Autodesk Inventor part; units mm, degrees
ref_plane "YZ Plane" through (0, 0, 0) normal (1, 0, 0) x (0, 1, 0)
ref_plane "XZ Plane" through (0, 0, 0) normal (0, 1, 0) x (-1, 0, 0)
ref_plane "XY Plane" through (0, 0, 0) normal (0, 0, 1) x (1, 0, 0)
sketch "Sketch1" plane through (0, 0, 0) normal (0, 0, 1) x (1, 0, 0)
  circle A0 centre (0, 0) radius 11.5
  circle A1 centre (0, 0) radius 1.65
  line L0 (-11.5, 0) -> (-11.5, -5)
  line L1 (-11.5, 0) -> (-11.5, 5)
  line L2 (-11.5, 5) -> (-10.3562, 5)
  line L3 (-11.5, -5) -> (-10.3562, -5)
  line L4 (11.5, 0) -> (11.5, 5)
  line L5 (11.5, 5) -> (10.3562, 5)
  line L6 (11.5, 0) -> (11.5, -5)
  line L7 (11.5, -5) -> (10.3562, -5)
  line L8 (-67.75, 0) -> (-67.75, 5)
  line L9 (-67.75, 5) -> (-11.5, 5)
  line L10 (-67.75, 0) -> (-67.75, -5)
  line L11 (-67.75, -5) -> (-11.5, -5)
  line L12 (67.75, -5) -> (67.75, 5)
  line L13 (67.75, 5) -> (11.5, 5)
  line L14 (11.5, -5) -> (67.75, -5)
  line L15 (67.75, -5) -> (71.75, -5)
  line L16 (71.75, -5) -> (71.75, 5)
  line L17 (71.75, 5) -> (67.75, 5)
  line L18 (-67.75, -5) -> (-71.75, -5)
  line L19 (-71.75, -5) -> (-71.75, 5)
  line L20 (-71.75, 5) -> (-67.75, 5)
  line L21 (0, 11.5) -> (-71.75, 11.5)
  line L22 (-71.75, 11.5) -> (-71.75, 5)
  line L23 (-71.75, -5) -> (-71.75, -11.5)
  line L24 (-71.75, -11.5) -> (0, -11.5)
  line L25 (0, -11.5) -> (71.75, -11.5)
  line L26 (71.75, -11.5) -> (71.75, -5)
  line L27 (71.75, 5) -> (71.75, 11.5)
  line L28 (0, 11.5) -> (71.75, 11.5)
  line L29 (67.75, 5) -> (67.75, 11.5)
  line L30 (67.75, 11.5) -> (63.75, 11.5)
  line L31 (63.75, 11.5) -> (63.75, -11.5)
  line L32 (-71.75, -11.5) -> (-63.75, -11.5)
  line L33 (-63.75, -11.5) -> (-63.75, 11.5)
  line L34 (-67.75, -11.5) -> (-75.75, -11.5)
  line L35 (-75.75, -11.5) -> (-75.75, 11.5)
  line L36 (-75.75, 11.5) -> (-67.75, 11.5)
  line L37 (-67.75, 11.5) -> (-67.75, -11.5)
  line L38 (67.75, 11.5) -> (75.75, 11.5)
  line L39 (75.75, 11.5) -> (75.75, -11.5)
  line L40 (75.75, -11.5) -> (67.75, -11.5)
  line L41 (67.75, -11.5) -> (67.75, 11.5)
  dimension "d0" = 23
  dimension "d1" = 3.3
  dimension "d4" = 5
  dimension "d5" = 5
  dimension "d6" = 5
  dimension "d7" = 5
  dimension "d12" = 4
  dimension "d13" = 4
  dimension "d20" = 4
  dimension "d21" = 8
  dimension "d24" = 8
  dimension "d25" = 8
extrude "Extrusion1" add sketch "Sketch1" along normal blind 8
extrude "Extrusion2" add sketch "Sketch1" against normal blind 80 contours L17 L16 L15 L12 | L29 L28 L27 L17 | L15 L26 L25 L41 | L37 L20 L22 L21 | L24 L23 L18 L37 | L27 L38 L39 L40 L26 L16 | L22 L19 L23 L34 L35 L36 | L8 L10 L18 L19 L20
sketch "Sketch4" plane through (75.75, -11.5, 8) normal (1, 0, 0) x (0, 0, -1)
  circle A0 centre (79.1099, 11.5) radius 1.75
  point P0 (8, 11.5)
  dimension "d26" = 3.5
extrude "Extrusion5" cut sketch "Sketch4" against normal blind 800
properties part number "Sensor houder" material "ABS Plastic"
Geometry check sheet. Reference: the model listing, model coordinates, mm. A direction names the side the tool comes from. Give positions to 0.01 mm unless a question says otherwise; leave off trailing zeros. Write each loop counter-clockwise with the first axis right and the second up, starting at its lowest first coordinate (ties: lowest second). Pieces come first, ordered by that corner, then holes. Notation, with made-up numbers: M -1.75,83 L 3.25,83 A25 ccw 3.25,119 Z; hole C 8,52.25 d1. An arc over 180 degrees is marked long. Answer as CSV lines item,"result". Start each with the question number.
Q1. Section check B-B, the plane x = 0. Record the cut outline in (y, z).
Q2. Section check A-A, the plane z = -63. Record the cut outline in (x, y).
Q3. Release check for a two-part mould opening along Y. For faces 3 (the face through (67.75, 0, -39)), 4 (the face through (0, -11.5, 3)), 5 (the face through (-71.69, 0.08, -69.36)) record: pulls with the +Y half, pulls with the -Y half, needs draft (parallel to the pull), parting line crosses it, or undercut.
Q4. Section check D-D, the plane y = -9.75. Record the cut outline in (x, z).
Q5. Go/stop test with flat-tipped pins: pin 1 (2 mm diameter, centred on y = 0, z = -71.11, fed in from +X); pin 2 (5 mm diameter, centred on x = -29.5, y = 2.5, fed in from -Z). Record where each tip stops, or that it passes through.
Q6. Material ranges on L1, parallel to X at y = 6.25, z = -37.5; L2, parallel to Y at x = 0, z = 6; L3, parallel to Z at x = -15, y = -2, recorded low to high.
Q7. Section check C-C, the plane y = 0. Record the cut outline in (x, z).
Q8. Tool access check on faces 1 (the face through (-72, 0, -80)), 2 (the face through (-1, 3, 0)). Record the directions out of +Z, -Z, +X, -X, +Y, -Y that give a thin tool (end or side, any length) a straight path to the whole face; none if there is none.
Geometry says:
1,outline,"M -11.5,0 L -1.65,0 L -1.65,8 L -11.5,8 Z; M 1.65,0 L 11.5,0 L 11.5,8 L 1.65,8 Z"
2,outline,"M -75.75,-11.5 L -67.75,-11.5 L -67.75,11.5 L -75.75,11.5 Z; M 67.75,-11.5 L 75.75,-11.5 L 75.75,11.5 L 67.75,11.5 Z"
3,face 3,"needs draft"
3,face 4,"pulls with the -Y half"
3,face 5,"undercut"
4,outline,"M -75.75,-80 L -67.75,-80 L -67.75,0 L 67.75,0 L 67.75,-80 L 75.75,-80 L 75.75,8 L -75.75,8 Z"
5,pin 1,"through"
5,pin 2,"z = 0"
6,L1,"-75.75 to -67.75, 67.75 to 75.75"
6,L2,"-11.5 to -1.65, 1.65 to 11.5"
6,L3,"0 to 8"
7,outline,"M -75.75,-80 L -67.75,-80 L -67.75,-72.86 L -75.75,-72.86 Z; M -75.75,-69.36 L -67.75,-69.36 L -67.75,0 L -1.65,0 L -1.65,8 L -75.75,8 Z; M 1.65,0 L 67.75,0 L 67.75,-69.36 L 75.75,-69.36 L 75.75,8 L 1.65,8 Z; M 67.75,-80 L 75.75,-80 L 75.75,-72.86 L 67.75,-72.86 Z"
8,face 1,"-Z, +X, -X, +Y, -Y"
8,face 2,"-Z, +Y, -Y"
